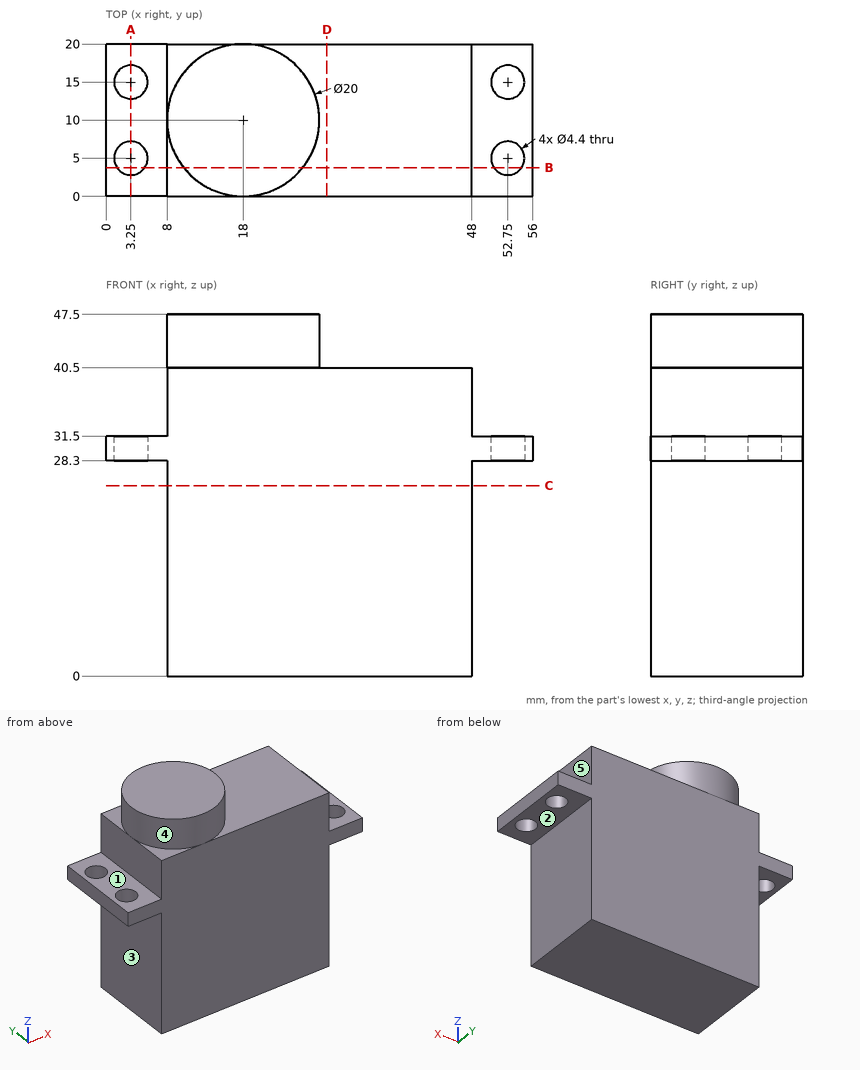
The drawing under review shows one solid part. Ordinate dimensions are in mm from its lowest x, y, z. A direction names the side the tool comes from. Coordinates: 2 decimals unless noted, no trailing zeros. Loops run counter-clockwise (first coordinate to the right, second up) from the corner with the lowest first, then second, coordinate; pieces in that order, holes last. Notation, with made-up numbers: M -30,74 L 25,74 A21 ccw 25,100 Z; hole C -5.75,78 d7. An arc over 180 degrees is marked long. Use one line per item in the form item = value.
(1) Consider section C-C (z = 25). Write out the cut boundary in (x, y).
Return value:
outline = M 8,0 L 48,0 L 48,20 L 8,20 Z
(2) Consider section B-B (y = 3.75). Write out the cut boundary in (x, z), and give its area (3 significant figures).
Return value:
outline = M 0,28.3 L 1.44,28.3 L 1.44,31.5 L 0,31.5 Z; M 5.06,28.3 L 8,28.3 L 8,0 L 48,0 L 48,28.3 L 50.94,28.3 L 50.94,31.5 L 48,31.5 L 48,40.5 L 25.81,40.5 L 25.81,47.5 L 10.19,47.5 L 10.19,40.5 L 8,40.5 L 8,31.5 L 5.06,31.5 Z; M 54.56,28.3 L 56,28.3 L 56,31.5 L 54.56,31.5 Z
area = 1,760 mm2
(3) For the marked faces 1, 2, 3, 4 and 5, list the 3-axis set-ups (+Z, -Z, +X, -X, +Y, -Y) from which the entire face can be reached by the end or side of a thin tool; tool diameter is ignored.
Return value:
face_1 = +Z, -X, +Y, -Y
face_2 = -Z, +X, +Y, -Y
face_3 = -Z, -X, +Y, -Y
face_4 = +Z
face_5 = +Z, +X, +Y, -Y
(4) Clearance check with flat-ended pins moving along their axes: P1, Ø1, axis at x = 31, y = 17, coming from the +Z side; P2, Ø2.5, axis at x = 50, y = 15, coming from the -Z side; P3, Ø4.5, axis at y = 12.5, z = 35, coming from the +X side; P4, Ø2.5, axis at x = 52.75, y = 5, coming from the -Z side. State where each tip first meets the part, or that it passes through.
Return value:
P1 = 40.5
P2 = 28.3
P3 = 48
P4 = through
(5) For line 1 along Y through (x, z) = (3.25, 29.95); line 2 along Y through (x, z) = (2, 28.5); line 3 along Z through (x, y) = (28, 12.5), list the stretches that pass through material, from the lowest coordinate up. Write a range as from..to.
Return value:
line_1 = 0..2.8, 7.2..12.8, 17.2..20
line_2 = 0..3.19, 6.81..13.19, 16.81..20
line_3 = 0..40.5
(6) Consider section D-D (x = 29). Write out the cut boundary in (y, z), and give its area (3 significant figures).
Return value:
outline = M 0,0 L 20,0 L 20,40.5 L 0,40.5 Z
area = 810 mm2
(7) Consider section A-A (x = 3.25). Write out the cut boundary in (y, z).
Return value:
outline = M 0,28.3 L 2.8,28.3 L 2.8,31.5 L 0,31.5 Z; M 7.2,28.3 L 12.8,28.3 L 12.8,31.5 L 7.2,31.5 Z; M 17.2,28.3 L 20,28.3 L 20,31.5 L 17.2,31.5 Z
